Could you check a few things on this model? Use its own coordinates, in mm. A direction names the side the tool comes from. Coordinates: 2 decimals unless noted, no trailing zeros. Loops run counter-clockwise (first coordinate to the right, second up) from the corner with the lowest first, then second, coordinate; pieces in that order, holes last. Notation, with made-up numbers: (-38, 72) -> (17, 72) arc R32 ccw to (17, 103) -> close; hole circle Ø4 at (47.5, 27.25). An arc over 180 degrees is marked (long way). One line per question, with ' | ' between items.
```python
from build123d import *

# Parameters (mm, degrees)
F0_R     = 152.4
F1_DEPTH = 38.1
F4_R     = 12.7
F5_DEPTH = 12.7


with BuildPart() as f1:
    # F0 (on Front) → F1 (new body)
    with BuildSketch(Plane.XZ):
        Circle(F0_R)
    extrude(amount=F1_DEPTH)

    # F2 (on Right) → F3 (revolve, cut)
    with BuildSketch(Plane.YZ):
        Polygon((-38.1, 152.908), (-38.1, 149.225), (-34.925, 149.225), (-34.925, 150.8125), (-31.75, 150.8125), (-31.75, 149.225), (-19.05, 149.225), (-19.05, 150.8125), (-5.591471, 150.8125), (-5.591471, 149.225), (0, 149.225), (0, 152.908), align=None)
    revolve(axis=Axis((0, -26.635785, 0), (0, -1, 0)), mode=Mode.SUBTRACT)

    # F4 (on face) → F5 (cut)
    with BuildSketch(Plane.XZ):
        Circle(F4_R)
    extrude(amount=F5_DEPTH, mode=Mode.SUBTRACT)


solid = f1.part
```
Q1. Imagine slicing it at D-D on z = 51. Write out the boundary of the cut face in (x, y) (3 decimals), plus the area to 3 significant figures.
Values follow:
outline: (-141.927, -34.925) -> (-140.239, -34.925) -> (-140.239, -38.1) -> (140.239, -38.1) -> (140.239, -34.925) -> (141.927, -34.925) -> (141.927, -31.75) -> (140.239, -31.75) -> (140.239, -19.05) -> (141.927, -19.05) -> (141.927, -5.591) -> (140.239, -5.591) -> (140.239, 0) -> (-140.239, 0) -> (-140.239, -5.591) -> (-141.927, -5.591) -> (-141.927, -19.05) -> (-140.239, -19.05) -> (-140.239, -31.75) -> (-141.927, -31.75) -> close | area: 10,700 mm2
Q2. We'd pull the mould along Y, two halves only. Please class faces 4 (the face through (-2, 0, -31)), 5 (the face through (-34, -34.925, 146)), 6 (the face through (-34, -19.05, 146)): released by +Y, released by -Y, zero draft, split by the parting line, or undercut.
Values follow:
face 4: released by +Y | face 5: released by -Y | face 6: undercut
Q3. Imagine slicing it at C-C on y = -27. Write out the boundary of the cut face in (x, z) (3 decimals).
Values follow:
outline: circle Ø298.45 at (0, 0)
Q4. For pin 1 (4 mm diameter, centred on x = 96.5, y = -17.5, fed in from -Z); pin 2 (1.5 mm diameter, centred on x = -24.5, y = -13, fed in from +Z); pin 3 (12.5 mm diameter, centred on x = -4.5, z = -1, fed in from +Y), each with a flat end and sliding along its axis, tell me the tip position at first contact or that it passes through.
Values follow:
pin 1: stops at z = -117.53 | pin 2: stops at z = 148.93 | pin 3: stops at y = -12.7
Q5. For faces 1 (the face through (90.8, -36.49, -118.42)), 2 (the face through (90.8, -2.76, -118.42)), 3 (the face through (90.8, -25.31, -118.42)), which set-ups out of +Z, -Z, +X, -X, +Y, -Y let a thin tool reach every point of the face, with its end or its side?
Values follow:
face 1: -Y | face 2: +Y | face 3: none
Q6. Please list where these lines run through material, in increasing order: L1, parallel to Z at x = 0, y = -6; L2, parallel to Y at x = -130, z = -74.5 (3 decimals); L3, parallel to X at y = -15, z = 3. Write a range as [from, to].
Values follow:
L1: z = [-150.81, -12.7], [12.7, 150.81] | L2: y = [-34.925, -31.75], [-19.05, -5.591] | L3: x = [-150.78, 150.78]
